Here's how the part is built. I have some questions about the finished solid (model axes, mm). Face numbers are marked on the shaded views. A direction names the side the tool comes from. Give positions to 0.01 mm unless a question says otherwise; leave off trailing zeros. Loops run counter-clockwise (first coordinate to the right, second up) from the corner with the lowest first, then second, coordinate; pieces in that order, holes last. Notation, with made-up numbers: (87.25, 8) - (137.25, 8) arc R20 cw to (137.25, 24) - close; hole circle Ø8 at (34.5, -7.5). An arc over 180 degrees is marked (long way). Return JSON: item names as keys, results as strings. Group by question number.
(1) On a 3-axis mill with a long thin cutter (end or side, diameter ignored), from which of +Z, -Z, +X, -X, +Y, -Y can I reach the whole of each face in a straight line? I mean the marked faces 4 and 5. Say none if no direction works.
(2) If we mould it in two halves opening along X, with no side actions, what happens to the marked faces 1, 2 and 3? For each: released by +X, released by -X, zero draft, split by the parting line, or undercut.
(3) If we section it at B-B (y = 14): Please give me the cut outline in (x, z), then the cut area to 3 significant figures.
(4) If we section it at C-C (x = -13): Please give me the cut outline in (y, z).
(5) If we section it at A-A (z = 49): Please give me the cut outline in (x, y), then the cut area to 4 significant figures.
(6) If we section it at D-D (z = 26): Please give me the cut outline in (x, y), then the cut area to 3 significant figures.
(7) I need wall thicknesses on probe 1 along X at (y, z) = (-20, 21.5); probe 2 along Y at (x, z) = (-26, 49); probe 3 along Z at (x, y) = (-17.5, 9). Which ranges of each line are inside material? Lowest first, please. Write a range as [from, to].
(8) For P1, Ø6, axis at x = 35.5, y = 3, coming from the +Z side; P2, Ø0.9, axis at x = 0.5, z = 52, coming from the -Y side; P3, Ø2.5, axis at x = -2.5, y = -23, coming from the +Z side, each with a flat end and sliding along its axis, tell me the tip position at first contact or that it passes through.
```python
from build123d import *

# Parameters (mm, degrees)
F0_W      = 90
F0_H      = 50
F1_DEPTH  = 50
F2_T      = -3
F4_DEPTH  = 90.001
F6_DEPTH  = 20
F7_W      = 7
F7_H      = 1
F7_W_2    = 1
F7_H_2    = 7
F8_DEPTH  = 3
F9_W      = 7.2
F9_H      = 1.2
F9_W_2    = 1.2
F9_H_2    = 7.2
F10_DEPTH = 3.5


with BuildPart() as f1:
    # F0 (on Top) → F1 (new body)
    with BuildSketch(Plane.XY):
        Rectangle(F0_W, F0_H)
    extrude(amount=F1_DEPTH)

    # F2
    f2_openings = [f1.faces().sort_by_distance(p)[0] for p in [
        (0, 0, 50),
    ]]
    offset(amount=F2_T, openings=f2_openings)

    # F3 (on face) → F4 (cut, through all)
    with BuildSketch(Plane(origin=(-45, 0, 0), x_dir=(0, -1, 0), z_dir=(-1, 0, 0))):
        Polygon((25, 30), (25, 50), (-5, 50), (10, 30), align=None)
    extrude(amount=-F4_DEPTH, mode=Mode.SUBTRACT)

    # F5 (on face) → F6 (cut)
    with BuildSketch(Plane.XY.offset(30)):
        Polygon((25, -22), (-25, -22), (-25, -23), (-23.6, -23), (-23.6, -24), (-25, -24), (-25, -25), (25, -25), (25, -24), (23.6, -24), (23.6, -23), (25, -23), align=None)
    extrude(amount=-F6_DEPTH, mode=Mode.SUBTRACT)

    # F7 (on face) → F8 (join)
    with BuildSketch(Plane.XY.offset(50)):
        with Locations((-27.5, 23.5)):
            Rectangle(F7_W, F7_H)
        with Locations((-43.5, 14.5)):
            Rectangle(F7_W_2, F7_H_2)
        with Locations((27.5, 23.5)):
            Rectangle(F7_W, F7_H)
        with Locations((43.5, 14.5)):
            Rectangle(F7_W_2, F7_H_2)
        with Locations((0, 23.5)):
            Rectangle(F7_W, F7_H)
    extrude(amount=F8_DEPTH)

    # F9 (on face) → F10 (cut)
    with BuildSketch(Plane(origin=(0, 0, 0), x_dir=(1, 0, 0), z_dir=(0, 0, -1))):
        with Locations((0, -23.5)):
            Rectangle(F9_W, F9_H)
        with Locations((27.5, -23.5)):
            Rectangle(F9_W, F9_H)
        with Locations((-27.5, -23.5)):
            Rectangle(F9_W, F9_H)
        with Locations((43.5, -14.5)):
            Rectangle(F9_W_2, F9_H_2)
        with Locations((-43.5, -14.5)):
            Rectangle(F9_W_2, F9_H_2)
    extrude(amount=-F10_DEPTH, mode=Mode.SUBTRACT)


solid = f1.part
```
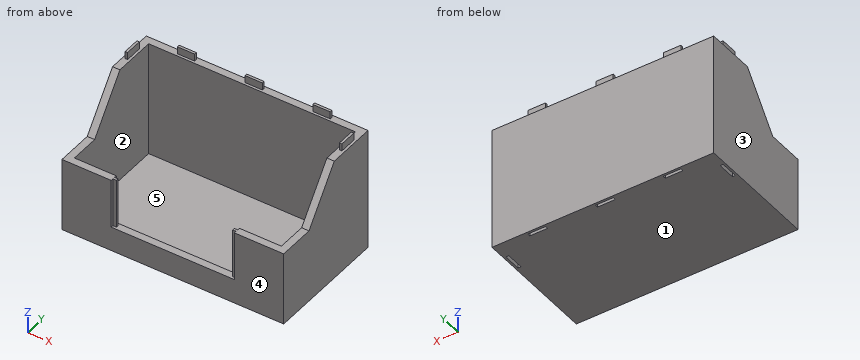
Values:
{
 "1": {"face 4": "+Z, -Z, +X, -X, -Y", "face 5": "+Z"},
 "2": {"face 1": "zero draft", "face 2": "undercut", "face 3": "released by -X"},
 "3": {"outline": "(-45, 0) - (-44.1, 0) - (-44.1, 3.5) - (-42.9, 3.5) - (-42.9, 0) - (42.9, 0) - (42.9, 3.5) - (44.1, 3.5) - (44.1, 0) - (45, 0) - (45, 50) - (44, 50) - (44, 53) - (43, 53) - (43, 50) - (42, 50) - (42, 3) - (-42, 3) - (-42, 50) - (-43, 50) - (-43, 53) - (-44, 53) - (-44, 50) - (-45, 50) - close", "area": "550 mm2"},
 "4": {"outline": "(-25, 0) - (25, 0) - (25, 50) - (22, 50) - (22, 3) - (-22, 3) - (-22, 10) - (-25, 10) - close"},
 "5": {"outline": "(-45, 4.25) - (-42, 4.25) - (-42, 22) - (42, 22) - (42, 4.25) - (45, 4.25) - (45, 25) - (-45, 25) - close", "area": "376.5 mm2"},
 "6": {"outline": "(-45, -25) - (-25, -25) - (-25, -24) - (-23.6, -24) - (-23.6, -23) - (-25, -23) - (-25, -22) - (-42, -22) - (-42, 22) - (42, 22) - (42, -22) - (25, -22) - (25, -23) - (23.6, -23) - (23.6, -24) - (25, -24) - (25, -25) - (45, -25) - (45, 25) - (-45, 25) - close", "area": "657 mm2"},
 "7": {"probe 1": "[-45, -42], [42, 45]", "probe 2": "[22, 25]", "probe 3": "[0, 3]"},
 "8": {"P1": "z = 3", "P2": "y = 23", "P3": "z = 10"}
}
